Read the model definition and answer for the solid it produces. Units are mm, in the model's axes. A direction names the side the tool comes from. Round coordinates to 2 decimals unless told otherwise and drop trailing zeros. Loops run counter-clockwise (first coordinate to the right, second up) from the corner with the lowest first, then second, coordinate; pieces in that order, holes last. Notation, with made-up numbers: (51, 70.5) -> (72, 70.5) arc R28 ccw to (72, 93.5) -> close; hole circle Ø6 at (-22, 79.5). An arc over 180 degrees is marked (long way). Put each result on its own line as item: value.
from build123d import *

# Parameters (mm, degrees)
SCHIZZO1_W                   = 120
SCHIZZO1_H                   = 70
ESTRUSIONE_ESTRUSIONE1_DEPTH = 5
SCHIZZO2_R                   = 4
ESTRUSIONE_ESTRUSIONE2_DEPTH = 20
SMUSSO1_SIZE                 = 2
SCHIZZO3_R                   = 0.95
TAGLIO_ESTRUSIONE1_DEPTH     = 15
RACCORDO1_R                  = 10
SCHIZZO4_R                   = 1.75
TAGLIO_ESTRUSIONE2_DEPTH     = 10


with BuildPart() as part:
    # Schizzo1 → Estrusione-Estrusione1 (new body)
    with BuildSketch(Plane.XY):
        Rectangle(SCHIZZO1_W, SCHIZZO1_H)
    extrude(amount=ESTRUSIONE_ESTRUSIONE1_DEPTH)

    # Schizzo2 → Estrusione-Estrusione2 (add)
    with BuildSketch(Plane.XY.offset(5)):
        with Locations((-50.15, 26.65)):
            Circle(SCHIZZO2_R)
        with Locations((50.15, -26.65)):
            Circle(SCHIZZO2_R)
        with Locations((50.15, 26.65)):
            Circle(SCHIZZO2_R)
        with Locations((-50.15, -26.65)):
            Circle(SCHIZZO2_R)
    extrude(amount=ESTRUSIONE_ESTRUSIONE2_DEPTH)

    # Smusso1
    smusso1_edges = [part.edges().sort_by_distance(p)[0] for p in [
        (-54.15, 26.65, 5),
        (46.15, -26.65, 5),
        (46.15, 26.65, 5),
        (-54.15, -26.65, 5),
    ]]
    chamfer(smusso1_edges, length=SMUSSO1_SIZE)

    # Schizzo3 → Taglio-Estrusione1 (cut)
    with BuildSketch(Plane.XY.offset(25)):
        with Locations((-50.15, 26.65)):
            Circle(SCHIZZO3_R)
        with Locations((50.15, 26.65)):
            Circle(SCHIZZO3_R)
        with Locations((50.15, -26.65)):
            Circle(SCHIZZO3_R)
        with Locations((-50.15, -26.65)):
            Circle(SCHIZZO3_R)
    extrude(amount=-TAGLIO_ESTRUSIONE1_DEPTH, mode=Mode.SUBTRACT)

    # Raccordo1
    raccordo1_edges = [part.edges().sort_by_distance(p)[0] for p in [
        (-60, 35, 2.5),
        (60, 35, 2.5),
        (60, -35, 2.5),
        (-60, -35, 2.5),
    ]]
    fillet(raccordo1_edges, radius=RACCORDO1_R)

    # Schizzo4 → Taglio-Estrusione2 (cut)
    with BuildSketch(Plane.XY.offset(5)):
        with Locations((-25, 21.101703565)):
            Circle(SCHIZZO4_R)
        with Locations((25, 21.101703565)):
            Circle(SCHIZZO4_R)
        with Locations((25, -21.101703565)):
            Circle(SCHIZZO4_R)
        with Locations((-25, -21.101703565)):
            Circle(SCHIZZO4_R)
    extrude(amount=-TAGLIO_ESTRUSIONE2_DEPTH, mode=Mode.SUBTRACT)


solid = part.part
Item 1: Find the intervals of material crossed by line 1 along Y through (x, z) = (-50.15, 14.25); line 2 along Y through (x, z) = (-25, 2.75); line 3 along Z through (x, y) = (0.5, -18), in increasing order.
Derived:
line 1: y = -30.65 to -27.6, -25.7 to -22.65, 22.65 to 25.7, 27.6 to 30.65
line 2: y = -35 to -22.85, -19.35 to 19.35, 22.85 to 35
line 3: z = 0 to 5
Item 2: Flat-ended cylindrical pins translate along their axes: pin 1 Ø2 at (x, z) = (-47, 15) entering from +Y; pin 2 Ø6 at (x, y) = (-13.5, 8.5) entering from +Z; pin 3 Ø0.6 at (x, y) = (50, 27) entering from +Z. Find the tip coordinate at first contact, or state that the pin passes through.
Derived:
pin 1: stops at y = 30.02
pin 2: stops at z = 5
pin 3: stops at z = 10
Item 3: The part is cut by section A-A (z = 15.5). Determine the outline of the cut face in (x, y).
Derived:
outline: circle Ø8 at (-50.15, -26.65); circle Ø8 at (-50.15, 26.65); circle Ø8 at (50.15, -26.65); circle Ø8 at (50.15, 26.65); hole circle Ø1.9 at (-50.15, -26.65); hole circle Ø1.9 at (-50.15, 26.65); hole circle Ø1.9 at (50.15, -26.65); hole circle Ø1.9 at (50.15, 26.65)
Item 4: Which of the six approach directions +Z, -Z, +X, -X, +Y, -Y give full straight-line access (tool end or side, diameter ignored) to faces 4 (the cylindrical face through (53.965, 27.851, 15.874)), 5 (the flat face through (60, 0, 2))?
Derived:
face 4: +Z
face 5: +Z, -Z, +X, +Y, -Y
Item 5: The part is cut by section C-C (y = 1). Determine the outline of the cut face in (x, z), then the cut area to 3 significant figures.
Derived:
outline: (-60, 0) -> (60, 0) -> (60, 5) -> (-60, 5) -> close
area: 600 mm^2
Item 6: For a pull along X with two mould halves and no side action, classify faces 1 (the cylindrical face through (-26.29, 22.284, 2.535)), 2 (the flat face through (-60, 0, 2)), 3 (the flat face through (51, -27.5, 25)) as pulls with the +X half, pulls with the -X half, needs draft (parallel to the pull), parting line crosses it, or undercut.
Derived:
face 1: undercut
face 2: pulls with the -X half
face 3: needs draft
Item 7: The part is cut by section B-B (x = 42.5). Determine the outline of the cut face in (y, z), then the cut area to 3 significant figures.
Derived:
outline: (-35, 0) -> (35, 0) -> (35, 5) -> (-35, 5) -> close
area: 350 mm^2
